from build123d import *

# Parameters (mm, degrees)
SKETCH011_W     = 126
SKETCH011_H     = 68
PAD006_DEPTH    = 3
SKETCH012_W     = 6
SKETCH012_H     = 12
PAD007_DEPTH    = 13.5
SKETCH013_R     = 2.25
POCKET004_DEPTH = 122.851
POCKET005_DEPTH = 3.5
CHAMFER004_SIZE = 1
CHAMFER005_SIZE = 1
CHAMFER008_SIZE = 1
SKETCH024_R     = 2.64
SKETCH024_R_2   = 8.15
SKETCH024_W     = 7.05
SKETCH024_H     = 19.25
POCKET012_DEPTH = 16.501
POCKET013_DEPTH = 1
CHAMFER010_SIZE = 2
SKETCH026_R     = 8.39
SKETCH026_R_2   = 6.64
POCKET014_DEPTH = 1.5
CHAMFER011_SIZE = 0.35
CHAMFER012_SIZE = 0.3
SKETCH030_R     = 5.14
SKETCH030_R_2   = 2.64
PAD012_DEPTH    = 4
SKETCH031_W     = 10.28
SKETCH031_H     = 2
POCKET016_DEPTH = 4
PAD016_DEPTH    = 4
FILLET004_R     = 0.1
SKETCH053_W     = 91
SKETCH053_H     = 2
POCKET028_DEPTH = 16.501
SKETCH054_W     = 11.6
SKETCH054_H     = 30.6
POCKET029_DEPTH = 16.501
SKETCH055_W     = 11.6
SKETCH055_H     = 36.6
POCKET030_DEPTH = 1.25


with BuildPart() as part:
    # Sketch011 → Pad006 (new body)
    with BuildSketch(Plane.XZ):
        with Locations((0, 34)):
            Rectangle(SKETCH011_W, SKETCH011_H)
    extrude(amount=PAD006_DEPTH)

    # Sketch012 (on Face5 of Pad006) → Pad007 (join)
    with BuildSketch(Plane(origin=(0, 0, 0), x_dir=(1, 0, 0), z_dir=(0, 1, 0))):
        with Locations((-56.85, -16)):
            Rectangle(SKETCH012_W, SKETCH012_H)
        with Locations((-56.85, -52)):
            Rectangle(SKETCH012_W, SKETCH012_H)
    pad007 = extrude(amount=PAD007_DEPTH)

    # Mirrored002: Pad007 across YZ
    add(pad007.mirror(Plane.YZ))

    # Sketch013 (on Face22 of Mirrored002) → Pocket004 (cut, through all)
    with BuildSketch(Plane(origin=(59.85, 0, 0), x_dir=(0, 0, 1), z_dir=(1, 0, 0))):
        with Locations((16, -7)):
            Circle(SKETCH013_R)
        with Locations((52, -7)):
            Circle(SKETCH013_R)
    extrude(amount=-POCKET004_DEPTH, mode=Mode.SUBTRACT)

    # Sketch014 (on Face10 of Pocket004) → Pocket005 (cut)
    with BuildSketch(Plane(origin=(-53.85, 0, 0), x_dir=(0, 0, 1), z_dir=(1, 0, 0))):
        Polygon((19.5, -9.020726), (19.5, -4.979274), (16, -2.958548), (12.5, -4.979274), (12.5, -9.020726), (16, -11.041452), align=None)
        Polygon((55.5, -9.020726), (55.5, -4.979274), (52, -2.958548), (48.5, -4.979274), (48.5, -9.020726), (52, -11.041452), align=None)
    pocket005 = extrude(amount=-POCKET005_DEPTH, mode=Mode.SUBTRACT)

    # Chamfer004
    chamfer004_edges = [part.edges().sort_by_distance(p)[0] for p in [
        (0, -3, 68),
        (63, -3, 34),
        (0, -3, 0),
        (-63, -3, 34),
    ]]
    chamfer(chamfer004_edges, length=CHAMFER004_SIZE)

    # Chamfer005
    chamfer005_edges = [part.edges().sort_by_distance(p)[0] for p in [
        (-63, -1, 68),
        (63, -1, 68),
    ]]
    chamfer(chamfer005_edges, length=CHAMFER005_SIZE)

    # Chamfer008
    chamfer008_edges = [part.edges().sort_by_distance(p)[0] for p in [
        (63, -1, 0),
        (-63, -1, 0),
    ]]
    chamfer(chamfer008_edges, length=CHAMFER008_SIZE)

    # Mirrored005: Pocket005 across YZ
    add(pocket005.mirror(Plane.YZ), mode=Mode.SUBTRACT)

    # Sketch024 (on Face62 of Mirrored005) → Pocket012 (cut, through all)
    with BuildSketch(Plane.XZ.offset(3)):
        with Locations((-12.4, 34)):
            Circle(SKETCH024_R)
        with Locations((37.2, 34)):
            Circle(SKETCH024_R_2)
        with Locations((-37.2, 34)):
            Rectangle(SKETCH024_W, SKETCH024_H)
    extrude(amount=-POCKET012_DEPTH, mode=Mode.SUBTRACT)

    # Sketch025 (on Face1 of Pocket012) → Pocket013 (cut)
    with BuildSketch(Plane(origin=(0, 0, 0), x_dir=(1, 0, 0), z_dir=(0, 1, 0))):
        Polygon((-40.725, -20.375), (-33.675, -20.375), (-33.675, -43.625), (-33.675, -47.625), (-40.725, -47.625), (-40.725, -24.375), align=None)
    extrude(amount=-POCKET013_DEPTH, mode=Mode.SUBTRACT)

    # Chamfer010
    chamfer010_edges = [part.edges().sort_by_distance(p)[0] for p in [
        (-15.04, -3, 34),
    ]]
    chamfer(chamfer010_edges, length=CHAMFER010_SIZE)

    # Sketch026 (on Face4 of Chamfer010) → Pocket014 (cut)
    with BuildSketch(Plane.XZ.offset(3)):
        with Locations((-12.4, 34)):
            Circle(SKETCH026_R)
        with Locations((-12.4, 34)):
            Circle(SKETCH026_R_2, mode=Mode.SUBTRACT)
    extrude(amount=-POCKET014_DEPTH, mode=Mode.SUBTRACT)

    # Chamfer011
    chamfer011_edges = [part.edges().sort_by_distance(p)[0] for p in [
        (-19.04, -3, 34),
        (-20.79, -3, 34),
    ]]
    chamfer(chamfer011_edges, length=CHAMFER011_SIZE)

    # Chamfer012
    chamfer012_edges = [part.edges().sort_by_distance(p)[0] for p in [
        (-37.2, -3, 24.375),
        (-40.725, -3, 34),
        (-33.675, -3, 34),
        (-37.2, -3, 43.625),
        (29.05, -3, 34),
    ]]
    chamfer(chamfer012_edges, length=CHAMFER012_SIZE)

    # Sketch030 (on Face3 of Chamfer012) → Pad012 (join)
    with BuildSketch(Plane(origin=(0, 0, 0), x_dir=(1, 0, 0), z_dir=(0, 1, 0))):
        with Locations((-12.4, -34)):
            Circle(SKETCH030_R)
        with Locations((-12.4, -34)):
            Circle(SKETCH030_R_2, mode=Mode.SUBTRACT)
    extrude(amount=PAD012_DEPTH)

    # Sketch031 (on Face83 of Pad012) → Pocket016 (cut)
    with BuildSketch(Plane(origin=(0, 4, 0), x_dir=(1, 0, 0), z_dir=(0, 1, 0))):
        with Locations((-12.4, -34)):
            Rectangle(SKETCH031_W, SKETCH031_H)
    extrude(amount=-POCKET016_DEPTH, mode=Mode.SUBTRACT)

    # Sketch035 (on Face3 of Pocket016) → Pad016 (join)
    with BuildSketch(Plane(origin=(0, 0, 0), x_dir=(1, 0, 0), z_dir=(0, 1, 0))):
        with BuildLine():
            ThreePointArc((-40, -53.5), (-41.5, -55), (-40, -56.5))
            Line((-40, -56.5), (40, -56.5))
            ThreePointArc((40, -56.5), (41.5, -55), (40, -53.5))
            Line((-40, -53.5), (40, -53.5))
        make_face()
        with BuildLine():
            ThreePointArc((-40, -10.5), (-41.5, -12), (-40, -13.5))
            Line((-40, -13.5), (40, -13.5))
            ThreePointArc((40, -13.5), (41.5, -12), (40, -10.5))
            Line((-40, -10.5), (40, -10.5))
        make_face()
    extrude(amount=PAD016_DEPTH)

    # Fillet004
    fillet004_edges = [part.edges().sort_by_distance(p)[0] for p in [
        (-18.69, -3, 34),
        (-17.04, -3, 34),
    ]]
    fillet(fillet004_edges, radius=FILLET004_R)

    # Sketch053 (on Face111 of Fillet004) → Pocket028 (cut, through all)
    with BuildSketch(Plane.XZ.offset(3)):
        with Locations((0, 67)):
            Rectangle(SKETCH053_W, SKETCH053_H)
    extrude(amount=-POCKET028_DEPTH, mode=Mode.SUBTRACT)

    # Sketch054 (on Face75 of Pocket028) → Pocket029 (cut, through all)
    with BuildSketch(Plane.XZ.offset(3)):
        with Locations((-37.2, 34)):
            Rectangle(SKETCH054_W, SKETCH054_H)
    extrude(amount=-POCKET029_DEPTH, mode=Mode.SUBTRACT)

    # Sketch055 (on Face21 of Pocket029) → Pocket030 (cut)
    with BuildSketch(Plane(origin=(0, 0, 0), x_dir=(1, 0, 0), z_dir=(0, 1, 0))):
        with Locations((-37.2, -34)):
            Rectangle(SKETCH055_W, SKETCH055_H)
    extrude(amount=-POCKET030_DEPTH, mode=Mode.SUBTRACT)


with BuildPart() as part_1:
    # Body004 placement: moved
    add(part.part.moved(Location((0, -66.95, 0))))


solid = part_1.part
Verification items for the finished model (mm, model axes). A direction names the side the tool comes from. Coordinates: 2 decimals unless noted, no trailing zeros. Order: outer loops, then holes, each group sorted by start corner. A loop starts at its lowest first (then second) coordinate and runs counter-clockwise, first axis right, second up. Notation, with made-up numbers: M 62,11 L 121,11 A29 cw 121,42 Z; hole C -39.5,33 d4. An arc over 180 degrees is marked long. One line per item, written item: value. Start each with the question number.
Item 1: Scan lines: probe 1 along Z at (x, y) = (-55.5, -60); probe 2 along Z at (x, y) = (59.1, -59.95); probe 3 along Y at (x, z) = (-59.1, 16). Record each from-to range of solid material in increasing order.
Item 2: Sectioned sample at A-A (x = 9). Enter the section's corners in (y, z).
Item 3: Gauge pin test, flat ends, axial feed: pin 1 (1 mm diameter, centred on x = 56, y = -59.5, fed in from +Z); pin 2 (1.8 mm diameter, centred on x = -56, y = -61.5, fed in from -Z); pin 3 (1.5 mm diameter, centred on x = -8, z = 11.5, fed in from +Y). Record the tip position at first contact, or that the pin passes through.
Item 4: Access from +Z, -Z, +X, -X, +Y, -Y to the whole of each face (thin tool, end or side, straight path). Record for faces 1 (the cylindrical face through (-11.18, -65.48, 36.34)), 2 (the flat face through (-57, -60, 46)), 3 (the flat face through (-55.576, -62.995, 50.274)), 4 (the flat face through (-57, -60, 10)), 5 (the flat face through (-1, -65, 56.5)).
Item 5: Mould release check, pull along Y, two halves, no side actions. Record for faces 6 (the flat face through (-1, -69.95, 34)), 7 (the flat face through (57, -60, 58)), 8 (the flat face through (57, -53.45, 16)), 9 (the flat face through (-57.35, -58, 50)): released by +Y, released by -Y, zero draft, split by the parting line, or undercut.
Item 6: Sectioned sample at B-B (y = -59.95). Count the separate pieces of the cut face and the enclosed holes in it, then the cut area to 3 significant figures.
Item 7: Sectioned sample at C-C (z = 61). Enter the section's corners in (x, y), then the cut area to 3 significant figures.
Conclusion:
1. probe 1: z = 10 to 12.5, 19.5 to 22, 46 to 48.5, 55.5 to 58
1. probe 2: z = 10 to 13.75, 18.25 to 22, 46 to 49.75, 54.25 to 58
1. probe 3: y = -69.95 to -62.2, -57.7 to -53.45
2. outline: M -69.95,1 L -68.95,0 L -66.95,0 L -66.95,10.5 L -62.95,10.5 L -62.95,13.5 L -66.95,13.5 L -66.95,53.5 L -62.95,53.5 L -62.95,56.5 L -66.95,56.5 L -66.95,66 L -69.95,66 Z
3. pin 1: stops at z = 58
3. pin 2: stops at z = 10
3. pin 3: stops at y = -62.95
4. face 1: +Y, -Y
4. face 2: +X, -X, +Y
4. face 3: none
4. face 4: -Z, +X, -X, +Y
4. face 5: +Z, +Y
5. face 6: released by -Y
5. face 7: zero draft
5. face 8: released by +Y
5. face 9: undercut
6. separate pieces: 8
6. enclosed holes: 0
6. area: 145 mm^2
7. outline: M -63,-68.95 L -62,-69.95 L 62,-69.95 L 63,-68.95 L 63,-66.95 L -63,-66.95 Z
7. area: 377 mm^2
